Design review of the part built by this model. Coordinates are the model's own, in mm. Face numbers are marked on the shaded views. A direction names the side the tool comes from. Give positions to 0.01 mm unless a question says otherwise; leave off trailing zeros. Loops run counter-clockwise (first coordinate to the right, second up) from the corner with the lowest first, then second, coordinate; pieces in that order, holes last.
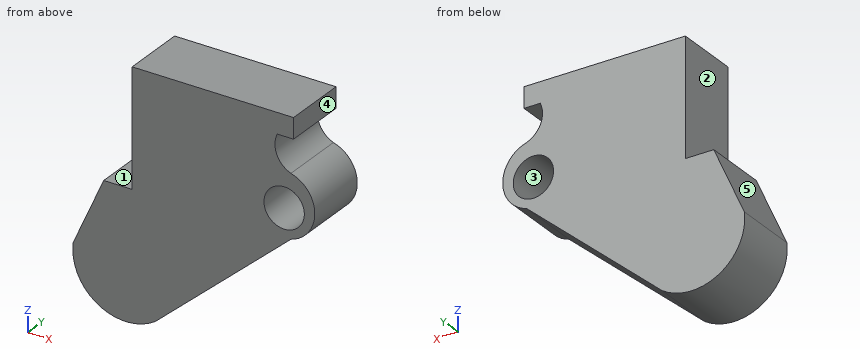
from build123d import *

# Parameters (mm, degrees)
F1_DEPTH = 2.54
F2_D     = 1.5875


# Not quite as in the source:
# - a feature names something its author has since deleted; it is built from what else it names


with BuildPart() as f1:
    # F0 (on Front) → F1 (new body)
    with BuildSketch(Plane.XZ):
        with BuildLine():
            Line((-49.06217859, 61.4019967616), (-49.06217859, 56.8155013025))
            Line((-49.06217859, 56.8155013025), (-42.814206332, 56.8155013025))
            ThreePointArc((-42.814206332, 56.8155013025), (-41.8729112238, 58.0492764711), (-42.814206332, 59.2830516398))
            ThreePointArc((-42.814206332, 59.2830516398), (-43.3685164044, 59.8206001728), (-43.3524362743, 60.592584312))
            Line((-43.3524362743, 60.592584312), (-42.7099727094, 60.592584312))
            Line((-42.7099727094, 60.592584312), (-42.7099727094, 61.4019967616))
            Line((-42.7099727094, 61.4019967616), (-49.06217859, 61.4019967616))
        make_face()
        with BuildLine():
            Line((-49.06217859, 56.8155013025), (-50.180206332, 56.8155013025))
            Line((-50.180206332, 56.8155013025), (-51.3855293393, 54.1270449758))
            ThreePointArc((-51.3855293393, 54.1270449758), (-50.3996469968, 52.1018542735), (-48.1477119029, 52.148219198))
            Line((-48.1477119029, 52.148219198), (-42.814206332, 56.8155013025))
            Line((-42.814206332, 56.8155013025), (-49.06217859, 56.8155013025))
        make_face()
    extrude(amount=F1_DEPTH)

    # F2 (through all)
    with Locations(Plane(origin=(0, 0, 0), x_dir=(1, 0, 0), z_dir=(0, 1, 0))):
        with Locations((-43.0801697075, -57.9093620181)):
            Hole(F2_D / 2)


solid = f1.part
Q1. Wall thickness on line 1 (Z direction, x = -43.25, y = -1.9); line 2 (X direction, y = -2.25, z = 58); line 3 (Z direction, x = -43.75, y = -0.4): over which ranges is each line inside the solid? List them lowest first.
Results:
line 1: z = 56.43 to 57.13, 58.68 to 59.61, 60.59 to 61.4
line 2: x = -49.06 to -43.87, -42.29 to -41.87
line 3: z = 56 to 57.48, 58.34 to 61.4
Q2. Take a section at C-C (x = -44.25). Give the boundary of the cut face in (y, z), plus the area to 3 significant figures.
Results:
outline: (-2.54, 55.56) - (0, 55.56) - (0, 61.4) - (-2.54, 61.4) - close
area: 14.8 mm2
Q3. Take a section at D-D (z = 53.25). Give the boundary of the cut face in (x, y), plus the area to 3 significant figures.
Results:
outline: (-51.3, -2.54) - (-46.89, -2.54) - (-46.89, 0) - (-51.3, 0) - close
area: 11.2 mm2
Q4. Draft analysis for pull direction X (two halves, no side actions). For the marked faces 1, 2 and 3, state which applies: pulls with the +X half, pulls with the -X half, needs draft (parallel to the pull), parting line crosses it, or undercut.
Results:
face 1: needs draft
face 2: pulls with the -X half
face 3: undercut
Q5. Tool access review of the marked faces 4 and 5: name each direction out of +Z, -Z, +X, -X, +Y, -Y from which nothing blocks a thin tool from reaching the whole face with its end or side.
Results:
face 4: +Z, +X, +Y, -Y
face 5: +Z, -X, +Y, -Y
Q6. Take a section at A-A (z = 58.5). Give the boundary of the cut face in (x, y), plus the area to 3 significant figures.
Results:
outline: (-49.06, -2.54) - (-43.61, -2.54) - (-43.61, 0) - (-49.06, 0) - close; (-42.55, -2.54) - (-41.95, -2.54) - (-41.95, 0) - (-42.55, 0) - close
area: 15.4 mm2
Q7. Take a section at B-B (y = -1.25). Give the boundary of the cut face in (x, z), plus the area to 3 significant figures.
Results:
outline: (-51.39, 54.13) arc R2.09 ccw to (-48.15, 52.15) - (-42.81, 56.82) arc R1.28 ccw to (-42.81, 59.28) arc R0.97 cw to (-43.35, 60.59) - (-42.71, 60.59) - (-42.71, 61.4) - (-49.06, 61.4) - (-49.06, 56.82) - (-50.18, 56.82) - close; hole circle Ø1.59 at (-43.08, 57.91)
area: 53.9 mm2
Q8. Insertion check: pin 1 (1.3 mm diameter, centred on y = -1, z = 58, fed in from -X); pin 2 (1 mm diameter, centred on x = -43.08, z = 57.91, fed in from -Y); pin 3 (0.6 mm diameter, centred on y = -1.5, z = 61, fed in from +X); pin 4 (0.7 mm diameter, centred on x = -43, y = -1, fed in from -Z). Each pin has a flat end and moves straight along its axis. Give the tip position at first contact, or say it passes through.
Results:
pin 1: stops at x = -49.06
pin 2: passes through
pin 3: stops at x = -42.71
pin 4: stops at z = 56.35
